Can you work these out from the model? Positions are in its coordinate system, mm. Round coordinates to 2 decimals unless told otherwise and drop trailing zeros. Loops run counter-clockwise (first coordinate to the right, second up) from the corner with the lowest first, then second, coordinate; pieces in that order, holes last. Notation, with made-up numbers: M 80.5,-30 L 129.5,-30 A22 cw 129.5,6 Z; hole C 12,-24 d2. An arc over 180 degrees is marked long. Answer as CSV lines item,"result".
from build123d import *

# Parameters (mm, degrees)
SKETCH1_R           = 2.0701
SKETCH1_R_2         = 14.2875
BOSS_EXTRUDE1_DEPTH = 2.286


with BuildPart() as part:
    # Sketch1 → Boss-Extrude1 (new body)
    with BuildSketch(Plane(origin=(0, 0, 0), x_dir=(-1, 0, 0), z_dir=(0, 0, -1))):
        Polygon((0, -23.114), (2.159, -25.273), (48.514, -25.273), (50.673, -23.114), (50.673, 23.114), (48.514, 25.273), (2.159, 25.273), (0, 23.114), (-2.159, 25.273), (-48.514, 25.273), (-50.673, 23.114), (-50.673, -23.114), (-48.514, -25.273), (-2.159, -25.273), align=None)
        with Locations((26.7081, -18.415)):
            Circle(SKETCH1_R, mode=Mode.SUBTRACT)
        with Locations((-45.1231, 0)):
            Circle(SKETCH1_R, mode=Mode.SUBTRACT)
        with Locations((26.7081, 18.415)):
            Circle(SKETCH1_R, mode=Mode.SUBTRACT)
        with Locations((-26.7081, 18.415)):
            Circle(SKETCH1_R, mode=Mode.SUBTRACT)
        with Locations((8.747587758, 17.960512242)):
            Circle(SKETCH1_R, mode=Mode.SUBTRACT)
        with Locations((44.668612242, 17.960512242)):
            Circle(SKETCH1_R, mode=Mode.SUBTRACT)
        with Locations((26.7081, 0)):
            Circle(SKETCH1_R_2, mode=Mode.SUBTRACT)
        with Locations((-44.668612242, -17.960512242)):
            Circle(SKETCH1_R, mode=Mode.SUBTRACT)
        with Locations((-8.747587758, 17.960512242)):
            Circle(SKETCH1_R, mode=Mode.SUBTRACT)
        with Locations((-26.7081, 0)):
            Circle(SKETCH1_R_2, mode=Mode.SUBTRACT)
        with Locations((-8.747587758, -17.960512242)):
            Circle(SKETCH1_R, mode=Mode.SUBTRACT)
        with Locations((-44.668612242, 17.960512242)):
            Circle(SKETCH1_R, mode=Mode.SUBTRACT)
        with Locations((44.668612242, -17.960512242)):
            Circle(SKETCH1_R, mode=Mode.SUBTRACT)
        with Locations((8.747587758, -17.960512242)):
            Circle(SKETCH1_R, mode=Mode.SUBTRACT)
        with Locations((-8.2931, 0)):
            Circle(SKETCH1_R, mode=Mode.SUBTRACT)
        with Locations((45.1231, 0)):
            Circle(SKETCH1_R, mode=Mode.SUBTRACT)
        with Locations((8.2931, 0)):
            Circle(SKETCH1_R, mode=Mode.SUBTRACT)
        with Locations((-26.7081, -18.415)):
            Circle(SKETCH1_R, mode=Mode.SUBTRACT)
    extrude(amount=-BOSS_EXTRUDE1_DEPTH)


solid = part.part
Item 1: If I drill on line 1 along Y through (x, z) = (-9.5, 0.4); line 2 along X through (y, z) = (8.5, 0.75); line 3 along X through (y, z) = (-7.5, 1.9), over which ranges is the centre line in solid material (lowest first)? Write a range as from..to.
Output:
line 1,"y = -25.27..-19.89, -16.03..-1.68, 1.68..16.03, 19.89..25.27"
line 2,"x = -50.67..-38.19, -15.22..15.22, 38.19..50.67"
line 3,"x = -50.67..-38.87, -14.55..14.55, 38.87..50.67"
Item 2: We'd pull the mould along Y, two halves only. Please class faces 1 (the face through (28.776, 18.506, 1.127)), 2 (the face through (-26, 25.273, 1)), 3 (the face through (1, 0, 2.286)), 4 (the face through (-1.064, -24.178, 1.127)): released by +Y, released by -Y, zero draft, split by the parting line, or undercut.
Output:
face 1,"undercut"
face 2,"released by +Y"
face 3,"zero draft"
face 4,"released by -Y"
Item 3: If we section it at B-B on y = -10.5: Write out the boundary of the cut face in (x, z).
Output:
outline,"M -50.67,0 L -36.4,0 L -36.4,2.29 L -50.67,2.29 Z; M -17.02,0 L 17.02,0 L 17.02,2.29 L -17.02,2.29 Z; M 36.4,0 L 50.67,0 L 50.67,2.29 L 36.4,2.29 Z"
Item 4: If we section it at A-A on y = 0: Write out the boundary of the cut face in (x, z), then the cut area to 3 significant figures.
Output:
outline,"M -50.67,0 L -47.19,0 L -47.19,2.29 L -50.67,2.29 Z; M -43.05,0 L -41,0 L -41,2.29 L -43.05,2.29 Z; M -12.42,0 L -10.36,0 L -10.36,2.29 L -12.42,2.29 Z; M -6.22,0 L 6.22,0 L 6.22,2.29 L -6.22,2.29 Z; M 10.36,0 L 12.42,0 L 12.42,2.29 L 10.36,2.29 Z; M 41,0 L 43.05,0 L 43.05,2.29 L 41,2.29 Z; M 47.19,0 L 50.67,0 L 50.67,2.29 L 47.19,2.29 Z"
area,"63.2 mm2"
Item 5: If we section it at C-C on z = 0.6: State how many separate pieces and enclosed holes the cut face has, then the cut area to 3 significant figures.
Output:
separate pieces,"1"
enclosed holes,"18"
area,"3,610 mm2"
